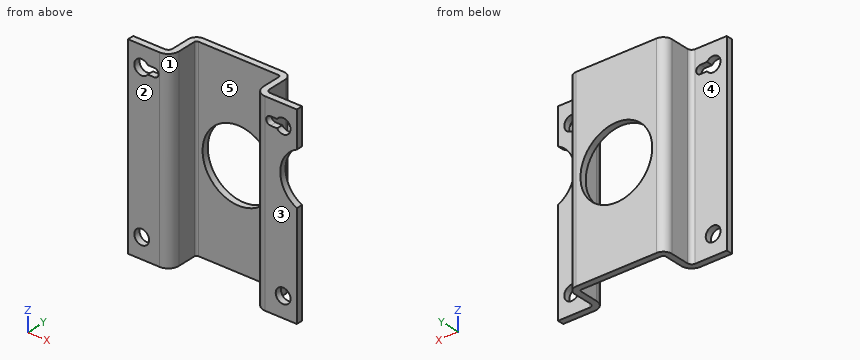
```python
from build123d import *

# Parameters (mm, degrees)
EXTRUDE_1_DEPTH     = 45.5
FILLET_1_R          = 4
FILLET_2_R          = 1
FILLET_3_R          = 5
FILLET_4_R          = 2
SKETCH_2_R          = 3.5
CUT_EXTRUDE_1_DEPTH = 10
SKETCH_3_R          = 13.760875338
CUT_EXTRUDE_2_DEPTH = 10
SKETCH_4_R          = 17
CUT_EXTRUDE_3_DEPTH = 10


with BuildPart() as part:
    # 草图1 → 凸台-拉伸1 (new, symmetric)
    with BuildSketch(Plane.XY):
        Polygon((0, 18), (-23, 18), (-23, 3), (-40, 3), (-40, 0), (-20, 0), (-20, 15), (0, 15), (20, 15), (20, 0), (40, 0), (40, 3), (23, 3), (23, 18), align=None)
    extrude(amount=EXTRUDE_1_DEPTH, both=True)

    # 圆角1
    fillet_1_edges = [part.edges().sort_by_distance(p)[0] for p in [
        (-23, 18, 0),
        (23, 18, 0),
    ]]
    fillet(fillet_1_edges, radius=FILLET_1_R)

    # 圆角2
    fillet_2_edges = [part.edges().sort_by_distance(p)[0] for p in [
        (-20, 15, 0),
        (20, 15, 0),
    ]]
    fillet(fillet_2_edges, radius=FILLET_2_R)

    # 圆角3
    fillet_3_edges = [part.edges().sort_by_distance(p)[0] for p in [
        (-20, 0, 0),
        (20, 0, 0),
    ]]
    fillet(fillet_3_edges, radius=FILLET_3_R)

    # 圆角4
    fillet_4_edges = [part.edges().sort_by_distance(p)[0] for p in [
        (-23, 3, 0),
        (23, 3, 0),
    ]]
    fillet(fillet_4_edges, radius=FILLET_4_R)

    # 草图2 → 切除-拉伸1 (cut)
    with BuildSketch(Plane.XZ):
        with Locations(Location((-33.5, -36, 0), (0, 0, 270))):
            Circle(SKETCH_2_R)
        with Locations(Location((33.5, -36, 0), (0, 0, 270))):
            Circle(SKETCH_2_R)
        with BuildLine():
            Line((-27.5, 38), (-30.627718677, 38))
            ThreePointArc((-30.627718677, 38), (-37, 36), (-30.627718677, 34))
            Line((-30.627718677, 34), (-27.5, 34))
            ThreePointArc((-27.5, 34), (-25.5, 36), (-27.5, 38))
        make_face()
        with BuildLine():
            Line((27.5, 34), (30.627718677, 34))
            ThreePointArc((30.627718677, 34), (37, 36), (30.627718677, 38))
            Line((30.627718677, 38), (27.5, 38))
            ThreePointArc((27.5, 38), (25.5, 36), (27.5, 34))
        make_face()
    extrude(amount=-CUT_EXTRUDE_1_DEPTH, mode=Mode.SUBTRACT)

    # 草图3 → 切除-拉伸2 (cut)
    with BuildSketch(Plane.XZ):
        with Locations((45.925407616, 16.065733646)):
            Circle(SKETCH_3_R)
    extrude(amount=-CUT_EXTRUDE_2_DEPTH, mode=Mode.SUBTRACT)

    # 草图4 → 切除-拉伸3 (cut)
    with BuildSketch(Plane(origin=(0, 18, 0), x_dir=(1, 0, 0), z_dir=(0, 1, 0))):
        with Locations(Location((0, 0, 0), (0, 0, 180))):
            Circle(SKETCH_4_R)
    extrude(amount=-CUT_EXTRUDE_3_DEPTH, mode=Mode.SUBTRACT)


solid = part.part
```
Check sheet for the modelled part. Datum: model origin and axes. Units: mm. Face numbers are marked on the shaded views. A direction names the side the tool comes from. Give positions to 0.01 mm unless a question says otherwise; leave off trailing zeros. Loops run counter-clockwise (first coordinate to the right, second up) from the corner with the lowest first, then second, coordinate; pieces in that order, holes last. Notation, with made-up numbers: M 46.5,-26 L 80.5,-26 A25 ccw 80.5,-10 Z; hole C 33.25,19 d6. An arc over 180 degrees is marked long. Answer in a Markdown table with one row per item.
1) Thickness scan on line 1 (Z direction, x = 0, y = 15.95); line 2 (X direction, y = 0.95, z = 36); line 3 (X direction, y = 0.85, z = 36). Record the ranges inside material, lowest first.
Solutions:
| item | result |
|---|---|
| line 1 | z = -45.5 to -17, 17 to 45.5 |
| line 2 | x = -40 to -37, -25.5 to -22.07, 22.07 to 25.5, 37 to 40 |
| line 3 | x = -40 to -37, -25.5 to -22.21, 22.21 to 25.5, 37 to 40 |
2) Cross-section at D-D (z = -36). Enter the section's corners in (x, y).
Solutions:
| item | result |
|---|---|
| outline | M -40,0 L -37,0 L -37,3 L -40,3 Z; M -30,0 L -25,0 A5 ccw -20,5 L -20,14 A1 cw -19,15 L 19,15 A1 cw 20,14 L 20,5 A5 ccw 25,0 L 30,0 L 30,3 L 25,3 A2 cw 23,5 L 23,14 A4 ccw 19,18 L -19,18 A4 ccw -23,14 L -23,5 A2 cw -25,3 L -30,3 Z; M 37,0 L 40,0 L 40,3 L 37,3 Z |
3) Cross-section at C-C (z = 0). Enter the section's corners in (x, y), plus the area to 3 significant figures.
Solutions:
| item | result |
|---|---|
| outline | M -40,0 L -25,0 A5 ccw -20,5 L -20,14 A1 cw -19,15 L -17,15 L -17,18 L -19,18 A4 ccw -23,14 L -23,5 A2 cw -25,3 L -40,3 Z; M 17,15 L 19,15 A1 cw 20,14 L 20,5 A5 ccw 25,0 L 40,0 L 40,3 L 25,3 A2 cw 23,5 L 23,14 A4 ccw 19,18 L 17,18 Z |
| area | 213 mm^2 |
4) Tool access check on the marked faces 3, 4 and 5. Record the directions out of +Z, -Z, +X, -X, +Y, -Y that give a thin tool (end or side, any length) a straight path to the whole face; none if there is none.
Solutions:
| item | result |
|---|---|
| face 3 | +Z, -Z, +X, -X, -Y |
| face 4 | +Z, -Z, -X, +Y |
| face 5 | +Z, -Z, -Y |
5) Depth check by flat-ended pin: pin 1 (2 mm diameter, centred on x = 5.5, z = -36, fed in from -Y); pin 2 (6 mm diameter, centred on y = 8, z = -11.5, fed in from +X); pin 3 (7 mm diameter, centred on y = 8.5, z = -11, fed in from -X); pin 4 (5.5 mm diameter, centred on x = -33.5, z = 36, fed in from -Y). Enter the tip coordinate at first touch or a pass-through.
Solutions:
| item | result |
|---|---|
| pin 1 | stops at y = 15 |
| pin 2 | stops at x = 23 |
| pin 3 | stops at x = -23 |
| pin 4 | passes through |
6) Cross-section at A-A (x = -33.5). Enter the section's corners in (y, z), plus the area to 3 significant figures.
Solutions:
| item | result |
|---|---|
| outline | M 0,-45.5 L 3,-45.5 L 3,-39.5 L 0,-39.5 Z; M 0,-32.5 L 3,-32.5 L 3,32.5 L 0,32.5 Z; M 0,39.5 L 3,39.5 L 3,45.5 L 0,45.5 Z |
| area | 231 mm^2 |
7) Cross-section at B-B (y = 1.5). Enter the section's corners in (x, z).
Solutions:
| item | result |
|---|---|
| outline | M -40,-45.5 L -21.43,-45.5 L -21.43,45.5 L -40,45.5 Z; M 21.43,-45.5 L 40,-45.5 L 40,3.65 A13.76 cw 40,28.49 L 40,45.5 L 21.43,45.5 Z; hole C -33.5,-36 d7; hole M -30.63,34 L -27.5,34 A2 ccw -27.5,38 L -30.63,38 A3.5 ccw long Z; hole M 27.5,34 L 30.63,34 A3.5 ccw long 30.63,38 L 27.5,38 A2 ccw Z; hole C 33.5,-36 d7 |
8) Mould release check, pull along X, two halves, no side actions. Record for the marked faces 1 and 2: released by +X, released by -X, zero draft, split by the parting line, or undercut.
Solutions:
| item | result |
|---|---|
| face 1 | undercut |
| face 2 | zero draft |
